Geometry check sheet. Reference: drawing and pictorial views, mm from the part's lowest x, y, z. A direction names the side the tool comes from. Round coordinates to 2 decimals unless told otherwise and drop trailing zeros. Write each loop counter-clockwise with the first axis right and the second up, starting at its lowest first coordinate (ties: lowest second). Pieces come first, ordered by that corner, then holes. Notation, with made-up numbers: M -21,9.25 L 2,9.25 A25 ccw 2,21.25 Z; hole C -14,-18 d8. An arc over 180 degrees is marked long. Answer in a Markdown table with one row per item.
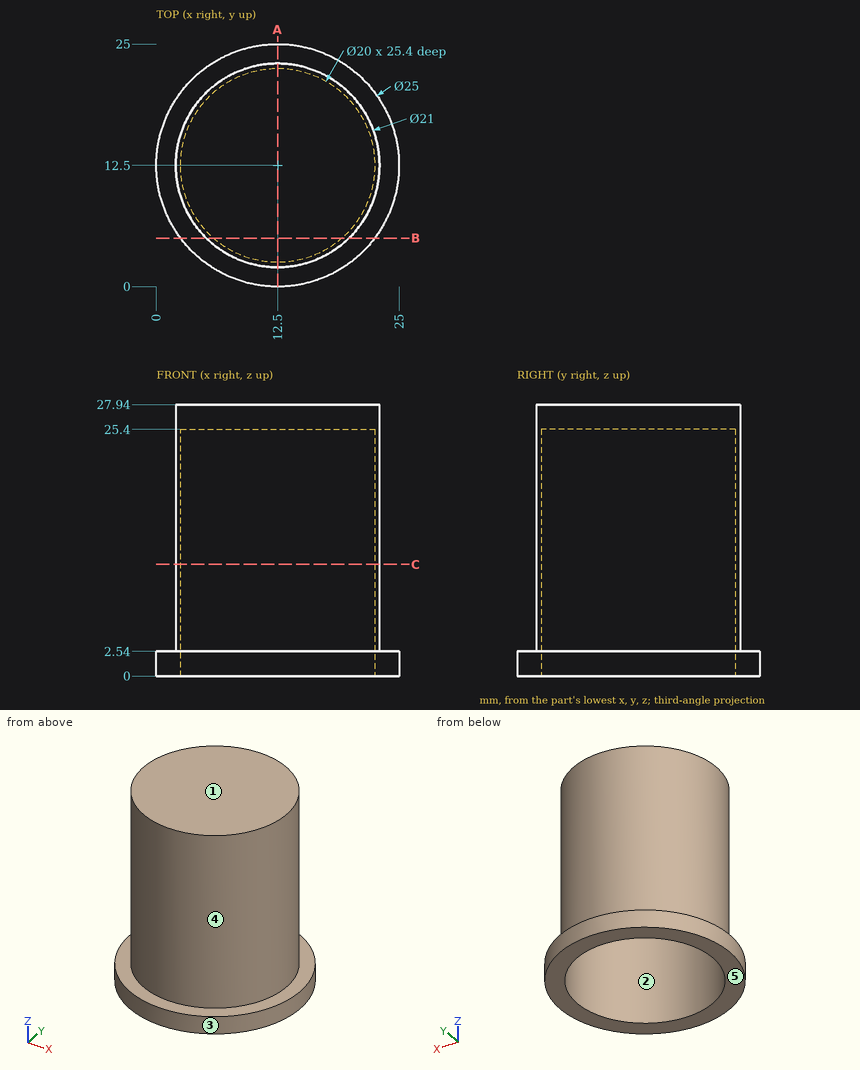
1. Scan lines: L1, parallel to Y at x = 12.5, z = 19.5; L2, parallel to Z at x = 22.25, y = 5.75; L3, parallel to X at y = 20.25, z = 23.75. Record each from-to range of solid material in increasing order.
Found:
| item | result |
|---|---|
| L1 | y = 2 to 2.5, 22.5 to 23 |
| L2 | z = 0 to 2.54 |
| L3 | x = 5.42 to 6.18, 18.82 to 19.58 |
2. Section check C-C, the plane z = 11.5. Record the cut outline in (x, y), and give its area (3 significant figures).
Found:
| item | result |
|---|---|
| outline | C 12.5,12.5 d21; hole C 12.5,12.5 d20 |
| area | 32.2 mm2 |
3. Section check B-B, the plane y = 5. Record the cut outline in (x, z), and give its area (3 significant figures).
Found:
| item | result |
|---|---|
| outline | M 2.5,0 L 5.89,0 L 5.89,25.4 L 19.11,25.4 L 19.11,0 L 22.5,0 L 22.5,2.54 L 19.85,2.54 L 19.85,27.94 L 5.15,27.94 L 5.15,2.54 L 2.5,2.54 Z |
| area | 88.1 mm2 |
4. Go/stop test with flat-tipped pins: pin 1 (4 mm diameter, centred on x = 8, z = 23, fed in from +Y); pin 2 (10 mm diameter, centred on x = 17, z = 21.5, fed in from -Y); pin 3 (12 mm diameter, centred on y = 10, z = 22.5, fed in from +X). Record where each tip stops, or that it passes through.
Found:
| item | result |
|---|---|
| pin 1 | stops at y = 22.7 |
| pin 2 | stops at y = 2 |
| pin 3 | stops at x = 23 |
5. Draft check along Y on the marked faces 1, 2 and 3. Enter one of: +Y half, -Y half, draft (parallel to the pull), parting line (faces both ways), or undercut.
Found:
| item | result |
|---|---|
| face 1 | draft |
| face 2 | undercut |
| face 3 | parting line |
6. Section check A-A, the plane x = 12.5. Record the cut outline in (y, z).
Found:
| item | result |
|---|---|
| outline | M 0,0 L 2.5,0 L 2.5,25.4 L 22.5,25.4 L 22.5,0 L 25,0 L 25,2.54 L 23,2.54 L 23,27.94 L 2,27.94 L 2,2.54 L 0,2.54 Z |
7. Access from +Z, -Z, +X, -X, +Y, -Y to the whole of each face (thin tool, end or side, straight path). Record for the marked faces 4 and 5.
Found:
| item | result |
|---|---|
| face 4 | +Z |
| face 5 | -Z, +X, -X, +Y, -Y |
